```python
from build123d import *

# Parameters (mm, degrees)
SKETCH1_R           = 17
SKETCH1_R_2         = 6
BOSS_EXTRUDE1_DEPTH = 5
SKETCH2_R           = 15
SKETCH2_R_2         = 13
BOSS_EXTRUDE2_DEPTH = 2.75
BOSS_EXTRUDE4_DEPTH = 5
SKETCH5_R           = 1
CUT_EXTRUDE1_DEPTH  = 20.5
SKETCH6_R           = 1.5
CUT_EXTRUDE2_DEPTH  = 8


with BuildPart() as part:
    # Sketch1 → Boss-Extrude1 (new body)
    with BuildSketch(Plane.XY):
        Circle(SKETCH1_R)
        Circle(SKETCH1_R_2, mode=Mode.SUBTRACT)
    extrude(amount=-BOSS_EXTRUDE1_DEPTH)

    # Sketch2 → Boss-Extrude2 (add)
    with BuildSketch(Plane.XY):
        Circle(SKETCH2_R)
        Circle(SKETCH2_R_2, mode=Mode.SUBTRACT)
    extrude(amount=BOSS_EXTRUDE2_DEPTH)

    # Sketch3 → Revolve1 (revolve)
    with BuildSketch(Plane(origin=(0, 0, 0), x_dir=(0, 0, -1), z_dir=(1, 0, 0))):
        Polygon((-2.75, 15), (0, 17), (0, 15), align=None)
    revolve(axis=Axis((0, 0, 0), (0, 0, 1)))

    # Sketch4 → Boss-Extrude4 (add)
    with BuildSketch(Plane(origin=(0, 0, -5), x_dir=(-1, 0, 0), z_dir=(0, 0, -1))):
        with BuildLine():
            Line((-14, 2.5), (-9, 2.5))
            Line((-9, 2.5), (-9, -2))
            ThreePointArc((-9, -2), (-9.146446609, -2.353553391), (-9.5, -2.5))
            Line((-9.5, -2.5), (-13.5, -2.5))
            ThreePointArc((-13.5, -2.5), (-13.853553391, -2.353553391), (-14, -2))
            Line((-14, -2), (-14, 2.5))
        make_face()
        with BuildLine():
            Line((13.5, -2.5), (9.5, -2.5))
            ThreePointArc((9.5, -2.5), (9.146446609, -2.353553391), (9, -2))
            Line((9, -2), (9, 2.5))
            Line((9, 2.5), (14, 2.5))
            Line((14, 2.5), (14, -2))
            ThreePointArc((14, -2), (13.853553391, -2.353553391), (13.5, -2.5))
        make_face()
    extrude(amount=BOSS_EXTRUDE4_DEPTH)

    # Sketch5 → Cut-Extrude1 (cut, through all)
    with BuildSketch(Plane(origin=(0, 2.5, 0), x_dir=(1, 0, 0), z_dir=(0, 1, 0))):
        with Locations((11.5, 7.5)):
            Circle(SKETCH5_R)
        with Locations((-11.5, 7.5)):
            Circle(SKETCH5_R)
    extrude(amount=-CUT_EXTRUDE1_DEPTH, mode=Mode.SUBTRACT)

    # Sketch6 → Cut-Extrude2 (cut)
    with BuildSketch(Plane(origin=(0, 0, -10), x_dir=(-1, 0, 0), z_dir=(0, 0, -1))):
        with Locations((-11.5, 0)):
            Circle(SKETCH6_R)
        with Locations((11.5, 0)):
            Circle(SKETCH6_R)
    extrude(amount=-CUT_EXTRUDE2_DEPTH, mode=Mode.SUBTRACT)


solid = part.part
```
Source: CAD feature listing. Evaluate the final solid. Frame: model axes, mm. A direction names the side the tool comes from. Give positions to 0.01 mm unless a question says otherwise; leave off trailing zeros. Loops run counter-clockwise (first coordinate to the right, second up) from the corner with the lowest first, then second, coordinate; pieces in that order, holes last. Notation, with made-up numbers: (-8, 55.25) -> (8, 55.25) arc R22 cw to (8, 61.25) -> close; hole circle Ø3 at (79.5, -4). An arc over 180 degrees is marked (long way). Use a Markdown table: item, result. Add a question column.
(1) Ray query, line 1 (X direction, y = -1.6, z = -7.5); line 2 (Y direction, x = -10.5, z = -8.5); line 3 (Y direction, x = 12, z = 2). Return the intervals inside material, ascending.
(2) Section query A-A (x = 0). Output: boundary loops of the cut face in (y, z).
(3) Access query for faces 4 (the face through (-10, 0, -6)), 5 (the face through (-9, 0, -7)), 6 (the face through (-10.316, -7.91, 1.356)), 7 (the face through (-10, 2.5, -7)), 8 (the face through (11, -2.5, -9)). Directions: +Z, -Z, +X, -X, +Y, -Y. A direction counts if a zero-diameter tool reaches every point of the face in a straight line with its end or side. Return the directions, or none.
(4) Section query C-C (z = -7.5). Output: boundary loops of the cut face in (x, y), then the cut area to 3 significant figures.
(5) Section query D-D (z = -1.5). Output: boundary loops of the cut face in (x, y), then the cut area to 3 significant figures.
(6) Pull-direction query (X, two-part tool) for faces 1 (the face through (-12, -2.5, -9)), 2 (the face through (12.454, 1.972, -7.8)), 3 (the face through (9.139, 14.334, -2.465)); classes: +X half, -X half, draft (parallel to the pull), parting line (faces both ways), or undercut.
(7) First-contact query: pin 1 Ø5 at (y, z) = (-7, -2) entering from -X; pin 2 Ø4 at (y, z) = (13, -4.5) entering from -X; pin 3 Ø0.9 at (x, y) = (11, 0.5) entering from -Z. Flat tips, straight axial feed; report the tip coordinate or a pass-through.
Checked values:
| question | item | result |
|---|---|---|
| 1 | line 1 | -14 to -12.5, -10.5 to -9, 9 to 10.5, 12.5 to 14 |
| 1 | line 2 | -2.5 to -1.12, 1.12 to 2.5 |
| 1 | line 3 | -9.88 to -5, 5 to 9.88 |
| 2 | outline | (-17, -5) -> (-6, -5) -> (-6, 0) -> (-13, 0) -> (-13, 2.75) -> (-15, 2.75) -> (-17, 0) -> close; (6, -5) -> (17, -5) -> (17, 0) -> (15, 2.75) -> (13, 2.75) -> (13, 0) -> (6, 0) -> close |
| 3 | face 4 | -Z |
| 3 | face 5 | -Z, +Y, -Y |
| 3 | face 6 | +Z |
| 3 | face 7 | -Z, +X, -X, +Y |
| 3 | face 8 | -Z, +X, -X, -Y |
| 4 | outline | (-14, -2) arc R0.5 ccw to (-13.5, -2.5) -> (-12.5, -2.5) -> (-12.5, -1.12) arc R1.5 cw to (-12.5, 1.12) -> (-12.5, 2.5) -> (-14, 2.5) -> close; (-10.5, -2.5) -> (-9.5, -2.5) arc R0.5 ccw to (-9, -2) -> (-9, 2.5) -> (-10.5, 2.5) -> (-10.5, 1.12) arc R1.5 cw to (-10.5, -1.12) -> close; (9, -2) arc R0.5 ccw to (9.5, -2.5) -> (10.5, -2.5) -> (10.5, -1.12) arc R1.5 cw to (10.5, 1.12) -> (10.5, 2.5) -> (9, 2.5) -> close; (12.5, -2.5) -> (13.5, -2.5) arc R0.5 ccw to (14, -2) -> (14, 2.5) -> (12.5, 2.5) -> (12.5, 1.12) arc R1.5 cw to (12.5, -1.12) -> close |
| 4 | area | 26.7 mm^2 |
| 5 | outline | circle Ø34 at (0, 0); hole circle Ø12 at (0, 0) |
| 5 | area | 795 mm^2 |
| 6 | face 1 | draft |
| 6 | face 2 | undercut |
| 6 | face 3 | parting line |
| 7 | pin 1 | x = -16.39 |
| 7 | pin 2 | x = -12.96 |
| 7 | pin 3 | z = -2 |
